For this review, take the finished solid that the model builds, in its own axes (mm). Face numbers are marked on the shaded views. A direction names the side the tool comes from. Coordinates: 2 decimals unless noted, no trailing zeros. Loops run counter-clockwise (first coordinate to the right, second up) from the corner with the lowest first, then second, coordinate; pieces in that order, holes last.
1. To check wall thickness, follow probe 1 along X at (y, z) = (-23, 0); probe 2 along Y at (x, z) = (-15, 49.5) (3 decimals); probe 3 along Z at (x, y) = (-25, 12). State the ranges of each line that lie inside material, in increasing order.
2. Take a section at C-C, the plane z = 43. State the section outline as (x, y) points (3 decimals), then the cut area to 3 significant figures.
3. Take a section at D-D, the plane y = 20.5. State the section outline as (x, z) points.
4. Take a section at A-A, the plane x = 0. State the section outline as (y, z) points (3 decimals).
5. Machinability: for the marked faces 4, 5 and 6, which of the approach directions +Z, -Z, +X, -X, +Y, -Y give a long, thin tool a straight path to every point of the face, cutting with its end or side? Answer none if there is none.
6. Clearance check with flat-ended pins moving along their axes: P1, Ø5, axis at y = 32.5, z = 22, coming from the -X side; P2, Ø4, axis at y = 7, z = -18, coming from the +X side; P3, Ø9.5, axis at y = 0, z = 0, coming from the -X side; P4, Ø5, axis at x = 53, y = -36, coming from the -Z side (3 decimals). State where each tip first meets the part, or that it passes through.
7. Mouldability with a two-part tool opening along Z and no side actions: class the marked faces 1, 2 and 3 as pulls with the +Z half, pulls with the -Z half, needs draft (parallel to the pull), parting line crosses it, or undercut.
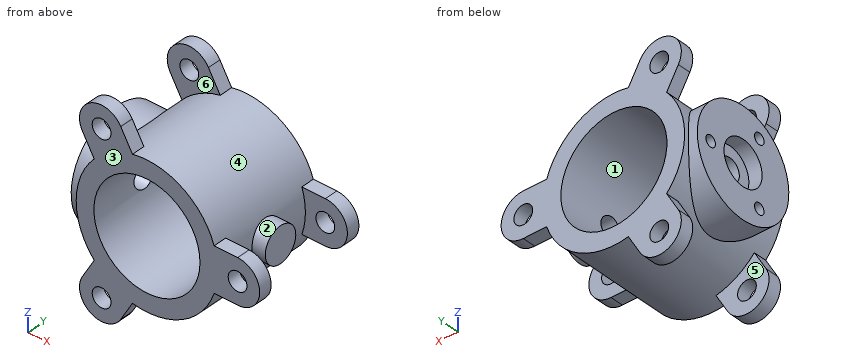
```python
from build123d import *

# Parameters (mm, degrees)
SKETCH1_R                   = 50.8
OUTSIDE_CYLINDER_DEPTH      = 41.275
BORE_START                  = -41.275
BORE_OUTLINE_R              = 38.1
BORE_DEPTH                  = 82.55
TAB_DEPTH                   = 9.525
TAB_HOLE_START              = 31.75
TAB_HOLE_OUTLINE_R          = 6.7437
TAB_HOLE_DEPTH              = 9.525
CIRPATTERN1_COUNT           = 3
MIRROR1_COPY_1_DEPTH        = 9.525
MIRROR1_COPY_2_DEPTH        = 9.525
MIRROR1_START               = 31.75
MIRROR1_COPY_3_SKETCH_R     = 6.7437
MIRROR1_COPY_3_DEPTH        = 9.525
MIRROR1_COPY_4_SKETCH_R     = 6.7437
MIRROR1_COPY_4_DEPTH        = 9.525
LEFT_PROTRUSION_REACH       = 163.254
LEFT_PROTRUSION_END_RADIUS  = 50.8
SKETCH5_R                   = 38.1
RIGHT_PROTRUSION_REACH      = 178.433
RIGHT_PROTRUSION_END_RADIUS = 50.8
RIGHT_START                 = 60.325
SKETCH6_R                   = 12.7
NARROW_START                = -57.15
NARROW_HOLE_OUTLINE_R       = 7.9375
NARROW_HOLE_DEPTH           = 114.3
SHALLOW_START               = -57.15
SHALLOW_HOLE_OUTLINE_R      = 15.875
SHALLOW_HOLE_OUTLINE_R_2    = 7.9375
SHALLOW_HOLE_DEPTH          = 9.525
CIRPATTERN2_COUNT           = 3


# Read off the part's stored shape, not the designer's step: Bore, Tab-hole, Narrow Hole, Shallow Hole
with BuildPart() as part:
    # Sketch1 → Outside Cylinder (new, symmetric)
    with BuildSketch(Plane(origin=(0, 0, 0), x_dir=(1, 0, 0), z_dir=(0, 1, 0))):
        with Locations(Location((0, 0, 0), (0, 0, 270))):
            Circle(SKETCH1_R)
    extrude(amount=OUTSIDE_CYLINDER_DEPTH, both=True)

    # Bore outline → Bore (cut)
    with BuildSketch(Plane(origin=(0, 0, 0), x_dir=(1, 0, 0), z_dir=(0, 1, 0)).offset(BORE_START)):
        Circle(BORE_OUTLINE_R)
    extrude(amount=BORE_DEPTH, mode=Mode.SUBTRACT)

    # Sketch3 → tab (add)
    with BuildSketch(Plane(origin=(0, 41.275, 0), x_dir=(1, 0, 0), z_dir=(0, 1, 0))):
        with BuildLine():
            Line((65.1002, 15.875), (48.255822188, 15.875))
            ThreePointArc((48.255822188, 15.875), (50.8, 0), (48.255822188, -15.875))
            Line((48.255822188, -15.875), (65.1002, -15.875))
            ThreePointArc((65.1002, -15.875), (80.9752, 0), (65.1002, 15.875))
        make_face()
    tab = extrude(amount=-TAB_DEPTH)

    # Tab-hole outline → Tab-hole (cut)
    with BuildSketch(Plane(origin=(0, 0, 0), x_dir=(1, 0, 0), z_dir=(0, 1, 0)).offset(TAB_HOLE_START)):
        with Locations((65.1002, 0)):
            Circle(TAB_HOLE_OUTLINE_R)
    tab_hole = extrude(amount=TAB_HOLE_DEPTH, mode=Mode.SUBTRACT)

    # CirPattern1: tab, Tab-hole ×3 about axis
    cirpattern1_axis = Axis((0, 0, 0), (0, 1, 0))
    add([tab.rotate(cirpattern1_axis, i * 360 / CIRPATTERN1_COUNT) for i in range(1, CIRPATTERN1_COUNT)])
    add([tab_hole.rotate(cirpattern1_axis, i * 360 / CIRPATTERN1_COUNT) for i in range(1, CIRPATTERN1_COUNT)], mode=Mode.SUBTRACT)

    # Mirror1: tab, Tab-hole across plane
    add(tab.mirror(Plane.ZX))
    add(tab_hole.mirror(Plane.ZX), mode=Mode.SUBTRACT)

    # Mirror1 copy 1 sketch → Mirror1 copy 1 (add)
    with BuildSketch(Plane(origin=(0, -41.275, 0), x_dir=(-0.4999999999999998, 0, -0.8660254037844387), z_dir=(0, -1, 0))):
        with BuildLine():
            Line((65.1002, -15.875), (48.255822188, -15.875))
            ThreePointArc((48.255822188, -15.875), (50.8, 0), (48.255822188, 15.875))
            Line((48.255822188, 15.875), (65.1002, 15.875))
            ThreePointArc((65.1002, 15.875), (80.9752, 0), (65.1002, -15.875))
        make_face()
    extrude(amount=-MIRROR1_COPY_1_DEPTH)

    # Mirror1 copy 2 sketch → Mirror1 copy 2 (add)
    with BuildSketch(Plane(origin=(0, -41.275, 0), x_dir=(-0.5000000000000004, 0, 0.8660254037844384), z_dir=(0, -1, 0))):
        with BuildLine():
            Line((65.1002, -15.875), (48.255822188, -15.875))
            ThreePointArc((48.255822188, -15.875), (50.8, 0), (48.255822188, 15.875))
            Line((48.255822188, 15.875), (65.1002, 15.875))
            ThreePointArc((65.1002, 15.875), (80.9752, 0), (65.1002, -15.875))
        make_face()
    extrude(amount=-MIRROR1_COPY_2_DEPTH)

    # Mirror1 copy 3 sketch → Mirror1 copy 3 (cut)
    with BuildSketch(Plane(origin=(0, 0, 0), x_dir=(-0.4999999999999998, 0, -0.8660254037844387), z_dir=(0, -1, 0)).offset(MIRROR1_START)):
        with Locations((65.1002, 0)):
            Circle(MIRROR1_COPY_3_SKETCH_R)
    extrude(amount=MIRROR1_COPY_3_DEPTH, mode=Mode.SUBTRACT)

    # Mirror1 copy 4 sketch → Mirror1 copy 4 (cut)
    with BuildSketch(Plane(origin=(0, 0, 0), x_dir=(-0.5000000000000004, 0, 0.8660254037844384), z_dir=(0, -1, 0)).offset(MIRROR1_START)):
        with Locations((65.1002, 0)):
            Circle(MIRROR1_COPY_4_SKETCH_R)
    extrude(amount=MIRROR1_COPY_4_DEPTH, mode=Mode.SUBTRACT)

    # Left Protrusion: up to this cylinder (the profile starts outside it)
    left_protrusion_end = Plane(origin=(0, 0, 0), z_dir=(0, -1, 0)) * Cylinder(LEFT_PROTRUSION_END_RADIUS, 429.108, mode=Mode.PRIVATE)
    # Sketch5 → Left Protrusion (add, up to the surface)
    with BuildSketch(Plane(origin=(-57.15, 0, 0), x_dir=(0, 0, -1), z_dir=(1, 0, 0)), mode=Mode.PRIVATE) as left_protrusion_sk1:
        with Locations(Location((0, 0, 0), (0, 0, 180))):
            Circle(SKETCH5_R)
    left_protrusion_tool1 = extrude(left_protrusion_sk1.sketch, amount=LEFT_PROTRUSION_REACH, mode=Mode.PRIVATE) - left_protrusion_end
    add(left_protrusion_tool1.solids().sort_by_distance((-57.15, 0, 0))[0])

    # Right Protrusion: up to this cylinder (the profile starts outside it)
    right_protrusion_end = Plane(origin=(0, 0, 0), z_dir=(0, -1, 0)) * Cylinder(RIGHT_PROTRUSION_END_RADIUS, 459.466, mode=Mode.PRIVATE)
    # Sketch6 → Right Protrusion (add, up to the surface)
    with BuildSketch(Plane(origin=(0, 0, 0), x_dir=(0, 0, -1), z_dir=(1, 0, 0)).offset(RIGHT_START), mode=Mode.PRIVATE) as right_protrusion_sk1:
        Circle(SKETCH6_R)
    right_protrusion_tool1 = extrude(right_protrusion_sk1.sketch, amount=-RIGHT_PROTRUSION_REACH, mode=Mode.PRIVATE) - right_protrusion_end
    add(right_protrusion_tool1.solids().sort_by_distance((60.325, 0, 0))[0])

    # Narrow Hole outline → Narrow Hole (cut)
    with BuildSketch(Plane.YZ.offset(NARROW_START)):
        Circle(NARROW_HOLE_OUTLINE_R)
    extrude(amount=NARROW_HOLE_DEPTH, mode=Mode.SUBTRACT)

    # Shallow Hole outline → Shallow Hole (cut)
    with BuildSketch(Plane.YZ.offset(SHALLOW_START)):
        Circle(SHALLOW_HOLE_OUTLINE_R)
        Circle(SHALLOW_HOLE_OUTLINE_R_2, mode=Mode.SUBTRACT)
    extrude(amount=SHALLOW_HOLE_DEPTH, mode=Mode.SUBTRACT)

    # Sketch13 → 3/8-16 Tapped Hole2 (revolve, cut)
    with BuildSketch(Plane(origin=(-57.15, -13.49502, 23.374060289), x_dir=(0, 0, 1), z_dir=(0, 1, 0))):
        Polygon((0, 0), (0, 17.624665582), (3.96875, 15.24), (3.96875, 0), align=None)
    f_3_8_16_tapped_hole2 = revolve(axis=Axis((-63.5, -13.49502, 23.374060289), (1, 0, 0)), mode=Mode.SUBTRACT)

    # CirPattern2: 3/8-16 Tapped Hole2 ×3 about axis
    cirpattern2_axis = Axis((0, 0, 0), (1, 0, 0))
    for i in range(1, CIRPATTERN2_COUNT):
        add(f_3_8_16_tapped_hole2.rotate(cirpattern2_axis, i * 360 / CIRPATTERN2_COUNT), mode=Mode.SUBTRACT)


solid = part.part
```
Results list:
1. probe 1: x = -57.15 to -38.1, 38.1 to 50.8
1. probe 2: y = -41.275 to -31.75, 31.75 to 41.275
1. probe 3: z = -44.22 to -28.75, 28.75 to 44.22
2. outline: (-43.157, -41.275) - (27.049, -41.275) - (27.049, 41.275) - (-43.157, 41.275) - (-43.157, 31.75) - (-27.049, 31.75) - (-27.049, -31.75) - (-43.157, -31.75) - close
2. area: 4,770 mm2
3. outline: (-57.15, -32.11) - (-39.36, -32.11) arc R50.8 ccw (long way) to (-39.36, 32.11) - (-57.15, 32.11) - close; hole circle Ø76.2 at (0, 0)
4. outline: (-41.275, -50.8) - (41.275, -50.8) - (41.275, -38.1) - (-41.275, -38.1) - close; (-41.275, 38.1) - (41.275, 38.1) - (41.275, 50.8) - (-41.275, 50.8) - close
5. face 4: none
5. face 5: -Z, -X
5. face 6: +Z, -X
6. P1: stops at x = -57.15
6. P2: stops at x = 48.21
6. P3: stops at x = 57.15
6. P4: stops at z = -15.875
7. face 1: undercut
7. face 2: parting line crosses it
7. face 3: needs draft
